Can you work these out from the model? Positions are in its coordinate system, mm. A direction names the side the tool comes from. Round coordinates to 2 decimals unless told otherwise and drop trailing zeros. Order: outer loops, then holes, each group sorted by start corner. A loop starts at its lowest first (then second) coordinate and runs counter-clockwise, first axis right, second up. Notation, with made-up numbers: M 50,88 L 107,88 A26 ccw 107,109 Z; hole C 13.5,-2 d11. An arc over 180 degrees is marked long. Answer as CSV lines item,"result". Start each with the question number.
from build123d import *

# Parameters (mm, degrees)
SKETCH1_R               = 10.668
SKETCH1_R_2             = 7.8994
MAINBODY_DEPTH          = 76.2
COAXENTRY_REACH         = 79.679
SKETCH2_W               = 25.4
SKETCH2_H               = 25.4
SKETCH3_R               = 1.524
ANTENNAMOUNTHOLES_DEPTH = 78.679163538


with BuildPart() as part:
    # Sketch1 → MainBody (new body)
    with BuildSketch(Plane(origin=(0, 0, 0), x_dir=(0, 0, -1), z_dir=(1, 0, 0))):
        with Locations(Location((0, 0, 0), (0, 0, 180))):
            Circle(SKETCH1_R)
        with Locations(Location((0, 0, 0), (0, 0, 180))):
            Circle(SKETCH1_R_2, mode=Mode.SUBTRACT)
    extrude(amount=MAINBODY_DEPTH)

    # Sketch2 → CoaxEntry (cut, up to next)
    with BuildSketch(Plane(origin=(0, 0, 0), x_dir=(1, 0, 0), z_dir=(0, 1, 0)), mode=Mode.PRIVATE) as coaxentry_sk1:
        with Locations((38.1, 0)):
            Rectangle(SKETCH2_W, SKETCH2_H)
    coaxentry_tool1 = extrude(coaxentry_sk1.sketch, amount=-COAXENTRY_REACH, mode=Mode.PRIVATE) & part.part
    add(coaxentry_tool1.solids().sort_by_distance((38.1, 0, 0))[0], mode=Mode.SUBTRACT)

    # Sketch3 → AntennaMountHoles (cut, through all)
    with BuildSketch(Plane(origin=(0, 0, 0), x_dir=(1, 0, 0), z_dir=(0, 1, 0))):
        with Locations(Location((4.7625, 0, 0), (0, 0, 90))):
            Circle(SKETCH3_R)
        with Locations(Location((17.4625, 0, 0), (0, 0, 90))):
            Circle(SKETCH3_R)
        with Locations(Location((71.4375, 0, 0), (0, 0, 90))):
            Circle(SKETCH3_R)
        with Locations(Location((58.7375, 0, 0), (0, 0, 90))):
            Circle(SKETCH3_R)
    extrude(amount=ANTENNAMOUNTHOLES_DEPTH, mode=Mode.SUBTRACT)


solid = part.part
(1) I want a section at A-A on z = 0. Write out the boundary of the cut face in (x, y).
(2) If I drill on line 1 along X through (y, z) = (8.95, 0); line 2 along Z through (x, y) = (29, 0.5); line 3 along Z through (x, y) = (51, -5.75), over which ranges is the centre line in solid material (lowest first)?
(3) I'm going to push flat-ended pins straight in: P1, Ø4, axis at x = 30, y = 6, coming from the -Z side; P2, Ø1.5, axis at x = 19, z = 8.5, coming from the -Y side; P3, Ø0.8, axis at x = 38, z = -9.5, coming from the -Y side; P4, Ø3, axis at y = -5.5, z = -2.5, coming from the +X side. Where does each tip first touch, or does it pass through?
(4) If we mould it in two halves opening along Z, with no side actions, what happens to faces 1 (the cylindrical face through (58.28, 9.188, -1.454)), 2 (the cylindrical face through (37.567, 7.008, 3.645)), 3 (the cylindrical face through (37.567, 9.464, 4.923)), 4 (the flat face through (38, 0, -9))? For each: +Z half, -Z half, draft (parallel to the pull), parting line (faces both ways), or undercut.
(5) I want a section at B-B on y = -8.75. Write out the boundary of the cut face in (x, z), and give its area (3 significant figures).
(6) For faces 5 (the flat face through (0, 4, -7)), 6 (the flat face through (38, 0, 9)), 7 (the cylindrical face through (70.98, 9.188, -1.454)), which set-ups out of +Z, -Z, +X, -X, +Y, -Y let a thin tool reach every point of the face, with its end or its side?
(7) I want a section at D-D on y = -4.5. Write out the boundary of the cut face in (x, z).
(8) I want a section at C-C on z = -3.25. Write out the boundary of the cut face in (x, y).
From the geometry:
1,outline,"M 0,-10.67 L 25.4,-10.67 L 25.4,-7.9 L 0,-7.9 Z; M 0,7.9 L 3.24,7.9 L 3.24,10.67 L 0,10.67 Z; M 6.29,7.9 L 15.94,7.9 L 15.94,10.67 L 6.29,10.67 Z; M 18.99,7.9 L 57.21,7.9 L 57.21,10.67 L 18.99,10.67 Z; M 50.8,-10.67 L 76.2,-10.67 L 76.2,-7.9 L 50.8,-7.9 Z; M 60.26,7.9 L 69.91,7.9 L 69.91,10.67 L 60.26,10.67 Z; M 72.96,7.9 L 76.2,7.9 L 76.2,10.67 L 72.96,10.67 Z"
2,line 1,"0 to 3.24, 6.29 to 15.94, 18.99 to 57.21, 60.26 to 69.91, 72.96 to 76.2"
2,line 2,"-10.66 to -7.88, 7.88 to 10.66"
2,line 3,"-8.99 to -5.42, 5.42 to 8.99"
3,P1,"z = -9.89"
3,P2,"y = -7.33"
3,P3,"y = 0"
3,P4,"through"
4,face 1,"undercut"
4,face 2,"undercut"
4,face 3,"parting line"
4,face 4,"draft"
5,outline,"M 0,-6.1 L 25.4,-6.1 L 25.4,6.1 L 0,6.1 Z; M 50.8,-6.1 L 76.2,-6.1 L 76.2,6.1 L 50.8,6.1 Z"
5,area,"620 mm²"
6,face 5,"+Z, -Z, -X, +Y, -Y"
6,face 6,"+Z, -Z, -Y"
6,face 7,"+Y"
7,outline,"M 0,-9.67 L 25.4,-9.67 L 25.4,-6.49 L 0,-6.49 Z; M 0,6.49 L 25.4,6.49 L 25.4,9.67 L 0,9.67 Z; M 50.8,-9.67 L 76.2,-9.67 L 76.2,-6.49 L 50.8,-6.49 Z; M 50.8,6.49 L 76.2,6.49 L 76.2,9.67 L 50.8,9.67 Z"
8,outline,"M 0,-10.16 L 25.4,-10.16 L 25.4,-7.2 L 0,-7.2 Z; M 0,7.2 L 76.2,7.2 L 76.2,10.16 L 0,10.16 Z; M 50.8,-10.16 L 76.2,-10.16 L 76.2,-7.2 L 50.8,-7.2 Z"
